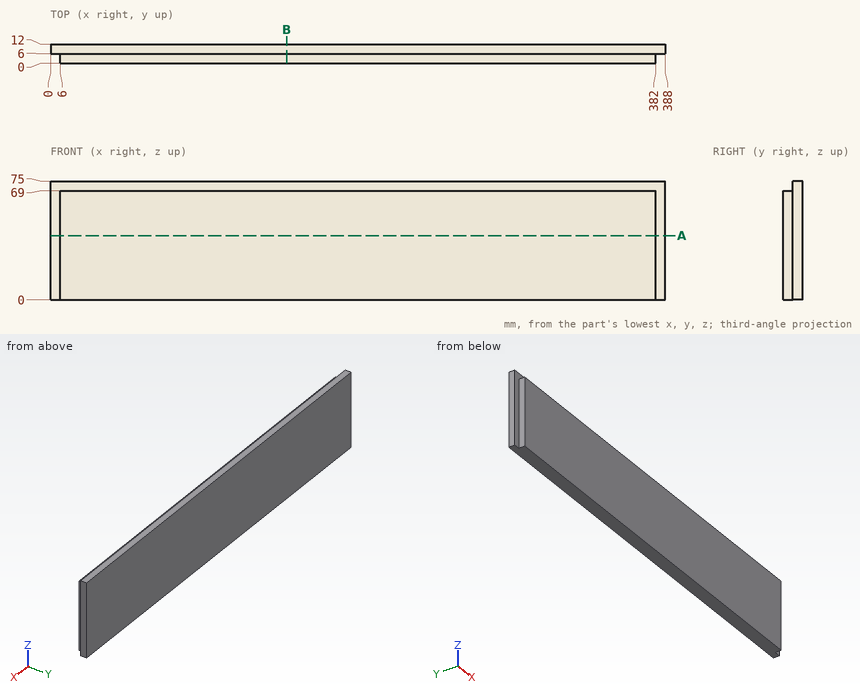
Geometry check sheet. Reference: drawing and pictorial views, mm from the part's lowest x, y, z. Give positions to 0.01 mm unless a question says otherwise; leave off trailing zeros. Write each loop counter-clockwise with the first axis right and the second up, starting at its lowest first coordinate (ties: lowest second). Pieces come first, ordered by that corner, then holes. Notation, with made-up numbers: M 53,-4.75 L 63,-4.75 A24 ccw 63,16.25 Z; hole C 59.25,41.5 d4. An arc over 180 degrees is marked long. Answer as CSV lines item,"result". Start each with the question number.
Q1. Go/stop test with flat-tipped pins: pin 1 (6 mm diameter, centred on x = 297, y = 5.5, fed in from -Z); pin 2 (3 mm diameter, centred on y = 2.5, z = 26.5, fed in from +X); pin 3 (3 mm diameter, centred on x = 199, y = 3, fed in from +Z). Record where each tip stops, or that it passes through.
Q2. Section check A-A, the plane z = 40.5. Record the cut outline in (x, y), then the cut area to 3 significant figures.
Q3. Material ranges on L1, parallel to X at y = 2.5, z = 37; L2, parallel to Z at x = 333, y = 4.75, recorded low to high.
Q4. Section check B-B, the plane x = 149. Record the cut outline in (y, z), then the cut area to 3 significant figures.
Geometry says:
1,pin 1,"z = 0"
1,pin 2,"x = 382"
1,pin 3,"z = 69"
2,outline,"M 0,6 L 6,6 L 6,0 L 382,0 L 382,6 L 388,6 L 388,12 L 0,12 Z"
2,area,"4,580 mm^2"
3,L1,"6 to 382"
3,L2,"0 to 69"
4,outline,"M 0,0 L 12,0 L 12,75 L 6,75 L 6,69 L 0,69 Z"
4,area,"864 mm^2"
